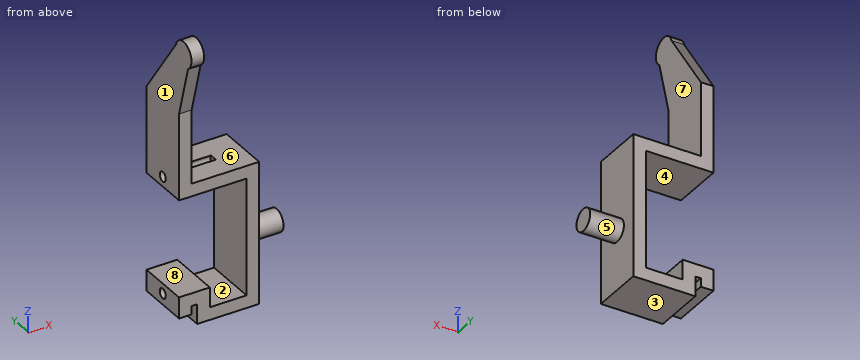
from build123d import *

# Parameters (mm, degrees)
EXTRUDE_1_DEPTH     = 12.5
SKETCH_2_R          = 1.15
CUT_EXTRUDE_1_DEPTH = 12
SKETCH_3_R          = 2.625
EXTRUDE_2_DEPTH     = 8
CUT_EXTRUDE_2_DEPTH = 8
EXTRUDE_3_DEPTH     = 3


with BuildPart() as part:
    # 草图1 → 凸台-拉伸1 (new body)
    with BuildSketch(Plane(origin=(0, 0, 0), x_dir=(1, 0, 0), z_dir=(0, 1, 0))):
        Polygon((0, 5), (0, 0), (7.3, 0), (7.3, 3), (7.3, 4.7), (16, 4.7), (16, 3), (16, 0), (16, -23), (0, -23), (0, -61), (3, -61), (3, -26), (19, -26), (19, 3), (19, 7.7), (4.3, 7.7), (4.3, 3), (3, 3), (3, 5), align=None)
    extrude(amount=EXTRUDE_1_DEPTH)

    # 草图2 → 切除-拉伸1 (cut)
    with BuildSketch(Plane.ZY):
        with Locations((-2.35, 6.25)):
            Circle(SKETCH_2_R)
        with Locations((25.35, 6.25)):
            Circle(SKETCH_2_R)
    extrude(amount=-CUT_EXTRUDE_1_DEPTH, mode=Mode.SUBTRACT)

    # 草图3 → 凸台-拉伸2 (add)
    with BuildSketch(Plane(origin=(19, 0, 0), x_dir=(0, 0, -1), z_dir=(1, 0, 0))):
        with Locations((-6.35, 6.25)):
            Circle(SKETCH_3_R)
    extrude(amount=EXTRUDE_2_DEPTH)

    # 草图4 → 切除-拉伸2 (cut)
    with BuildSketch(Plane(origin=(3, 0, 0), x_dir=(0, 0, -1), z_dir=(1, 0, 0))):
        with BuildLine():
            Line((-61, 12.5), (-61, 0))
            ThreePointArc((-61, 0), (-60.261770725, 0.750275482), (-59.312624964, 1.205267883))
            Line((-59.312624964, 1.205267883), (-43.5, 12.5))
            Line((-43.5, 12.5), (-61, 12.5))
        make_face()
    extrude(amount=-CUT_EXTRUDE_2_DEPTH, mode=Mode.SUBTRACT)

    # 草图4<4> → 凸台-拉伸3 (add)
    with BuildSketch(Plane(origin=(3, 0, 0), x_dir=(0, 0, -1), z_dir=(1, 0, 0))):
        with BuildLine():
            ThreePointArc((-61, 0), (-60.221329006, -4.246956372), (-55.974372634, -3.468285379))
            Line((-55.974372634, -3.468285379), (-43.5, 0))
            Line((-43.5, 0), (-61, 0))
        make_face()
    extrude(amount=-EXTRUDE_3_DEPTH)


solid = part.part
The listing builds one solid part. Answer for the finished solid, in the listing's coordinates (mm). Face numbers are marked on the shaded views. A direction names the side the tool comes from. Round coordinates to 2 decimals unless told otherwise and drop trailing zeros. Order: outer loops, then holes, each group sorted by start corner. A loop starts at its lowest first (then second) coordinate and runs counter-clockwise, first axis right, second up. Notation, with made-up numbers: (6.25, 16) - (48.25, 16) arc R8 ccw to (48.25, 29) - close; hole circle Ø6 at (-23.5, 18). An arc over 180 degrees is marked (long way). Write item = value, one per line. Start each with the question number.
1) Straight lines are drawn through the part: L1, parallel to Z at x = 5, y = 6.25; L2, parallel to Y at x = 7.5, z = 25.35; L3, parallel to Z at x = 7.5, y = 6.25. For each, find the intervals that lie inside material, in ascending order.
2) Given pin 1 (3.5 mm diameter, centred on x = 1.5, y = 7, fed in from -Z); pin 2 (2.5 mm diameter, centred on y = 6.25, z = -2.35, fed in from +X); pin 3 (2.5 mm diameter, centred on x = 11, y = 5, fed in from +Z), each flat-ended and moving along its own axis, determine where each tip first touches the part or whether it passes through.
3) Section A-A, the plane z = -2.35 is taken. Write down the section's boundary in (x, y), plus the area to 3 significant figures.
4) Section B-B, the plane x = 14.25 is taken. Write down the section's boundary in (y, z), plus the area to 3 significant figures.
5) For a pull along Z with two mould halves and no side action, classify the marked faces 6, 7 and 8 as released by +Z, released by -Z, zero draft, split by the parting line, or undercut.
6) Section C-C, the plane y = 6.25 is taken. Write down the section's boundary in (x, z) (3 decimals), plus the area to 3 significant figures.
7) For the marked faces 1, 2, 3, 4 and 5, determine the directions among +Z, -Z, +X, -X, +Y, -Y from which every point of the face is accessible in a straight line to the end or side of a thin tool.
8) Section D-D, the plane y = 10.5 is taken. Write down the section's boundary in (x, z).
Results list:
q1.L1 = -7.7 to -3.5, -1.2 to 0, 23 to 24.2
q1.L2 = 0 to 5.1, 7.4 to 12.5
q1.L3 = -7.7 to -4.7, 23 to 24.2
q2.pin_1 = -5
q2.pin_2 = 19
q2.pin_3 = 26
q3.outline = (0, 0) - (7.3, 0) - (7.3, 5.1) - (0, 5.1) - close; (0, 7.4) - (7.3, 7.4) - (7.3, 12.5) - (0, 12.5) - close; (16, 0) - (19, 0) - (19, 12.5) - (16, 12.5) - close
q3.area = 112 mm^2
q4.outline = (0, -7.7) - (12.5, -7.7) - (12.5, -4.7) - (0, -4.7) - close; (0, 23) - (12.5, 23) - (12.5, 26) - (0, 26) - close
q4.area = 75.0 mm^2
q5.face_6 = released by +Z
q5.face_7 = zero draft
q5.face_8 = undercut
q6.outline = (0, -5) - (3, -5) - (3, -3.5) - (0, -3.5) - close; (0, -1.2) - (7.3, -1.2) - (7.3, 0) - (0, 0) - close; (0, 23) - (16, 23) - (16, -4.7) - (7.3, -4.7) - (7.3, -3.5) - (4.3, -3.5) - (4.3, -7.7) - (19, -7.7) - (19, 3.725) - (27, 3.725) - (27, 8.975) - (19, 8.975) - (19, 26) - (12, 26) - (12, 24.2) - (0, 24.2) - close; (0, 26.5) - (3, 26.5) - (3, 52.25) - (0, 52.25) - close
q6.area = 299 mm^2
q7.face_1 = +Z, -Z, -X, +Y, -Y
q7.face_2 = +Y, -Y
q7.face_3 = -Z, +X, -X, +Y, -Y
q7.face_4 = -X, +Y, -Y
q7.face_5 = +X
q8.outline = (0, -5) - (3, -5) - (3, -3) - (4.3, -3) - (4.3, -7.7) - (19, -7.7) - (19, 26) - (3, 26) - (3, 46.3) - (0, 46.3) - (0, 23) - (16, 23) - (16, -4.7) - (7.3, -4.7) - (7.3, 0) - (0, 0) - close
